```python
from build123d import *

# Parameters (mm, degrees)
F0_W     = 12
F0_H     = 12
F1_DEPTH = 15
F2_R     = 3.5
F3_DEPTH = 4
F4_R     = 2.65
F5_DEPTH = 20


with BuildPart() as f1:
    # F0 (on Right) → F1 (new body)
    with BuildSketch(Plane.YZ):
        Rectangle(F0_W, F0_H)
    extrude(amount=F1_DEPTH)

    # F2 (on face) → F3 (cut)
    with BuildSketch(Plane(origin=(0, 6, 0), x_dir=(-1, 0, 0), z_dir=(0, 1, 0))):
        with Locations((-10.337353, 0)):
            Circle(F2_R)
    extrude(amount=-F3_DEPTH, mode=Mode.SUBTRACT)

    # F4 (on face) → F5 (cut)
    with BuildSketch(Plane(origin=(0, 2, 0), x_dir=(-1, 0, 0), z_dir=(0, 1, 0))):
        with Locations((-10.337353, 0)):
            Circle(F4_R)
    extrude(amount=-F5_DEPTH, mode=Mode.SUBTRACT)


solid = f1.part
```
Check sheet for the modelled part. Datum: model origin and axes. Units: mm. A direction names the side the tool comes from. Round coordinates to 2 decimals unless told otherwise and drop trailing zeros. Order: outer loops, then holes, each group sorted by start corner. A loop starts at its lowest first (then second) coordinate and runs counter-clockwise, first axis right, second up.
1) Section check C-C (x = 11.75). Record the boundary of the cut face in (y, z), and give its area (3 significant figures).
2) Go/stop test with flat-tipped pins: pin 1 Ø2 at (x, z) = (8.5, -1.5) entering from +Y; pin 2 Ø1 at (x, z) = (11, 0.5) entering from +Y. Record where each tip stops, or that it passes through.
3) Section check D-D (x = 13.25). Record the boundary of the cut face in (y, z).
4) Tool access check on faces 5 (the flat face through (15, 0, 0)), 6 (the cylindrical face through (13.834, 4.028, 0.154)). Record the directions out of +Z, -Z, +X, -X, +Y, -Y that give a thin tool (end or side, any length) a straight path to the whole face; none if there is none.
5) Section check A-A (z = 0). Record the boundary of the cut face in (x, y), and give its area (3 significant figures).
6) Mould release check, pull along Z, two halves, no side actions. Record for faces 1 (the flat face through (7, 0, 6)), 2 (the flat face through (7, 0, -6)), 3 (the cylindrical face through (7.889, -1.944, -1.015)), 4 (the flat face through (0, 0, 0)): +Z half, -Z half, draft (parallel to the pull), parting line (faces both ways), or undercut.
7) Section check B-B (y = 2.5). Record the boundary of the cut face in (x, z).
8) Scan lines: line 1 (Z direction, x = 10.25, y = 5.75); line 2 (Y direction, x = 9.5, z = 3); line 3 (Z direction, x = 12, y = -3). Record each from-to range of solid material in increasing order.
Result:
1. outline: (-6, -6) - (6, -6) - (6, -3.2) - (2, -3.2) - (2, -2.24) - (-6, -2.24) - close; (-6, 2.24) - (2, 2.24) - (2, 3.2) - (6, 3.2) - (6, 6) - (-6, 6) - close
1. area: 82.5 mm2
2. pin 1: stops at y = 2
2. pin 2: passes through
3. outline: (-6, -6) - (6, -6) - (6, -1.94) - (2, -1.94) - (2, 1.94) - (6, 1.94) - (6, 6) - (-6, 6) - close
4. face 5: +Z, -Z, +X, +Y, -Y
4. face 6: +Y
5. outline: (0, -6) - (7.69, -6) - (7.69, 2) - (6.84, 2) - (6.84, 6) - (0, 6) - close; (12.99, -6) - (15, -6) - (15, 6) - (13.84, 6) - (13.84, 2) - (12.99, 2) - close
5. area: 110 mm2
6. face 1: +Z half
6. face 2: -Z half
6. face 3: undercut
6. face 4: draft
7. outline: (0, -6) - (15, -6) - (15, 6) - (0, 6) - close; hole circle Ø7 at (10.34, 0)
8. line 1: z = -6 to -3.5, 3.5 to 6
8. line 2: y = -6 to 2
8. line 3: z = -6 to -2.06, 2.06 to 6
